Can you work these out from the drawing? Everything is in mm from the part's minimum corner. A direction names the side the tool comes from. Give positions to 0.01 mm unless a question says otherwise; leave off trailing zeros. Write each loop counter-clockwise with the first axis right and the second up, starting at its lowest first coordinate (ties: lowest second). Pieces come first, ordered by that corner, then holes. Notation, with made-up numbers: M 13,42.25 L 39,42.25 A30 ccw 39,77.25 Z; hole C -28,10.25 d7. An arc over 180 degrees is marked long. One line per item, written item: value.
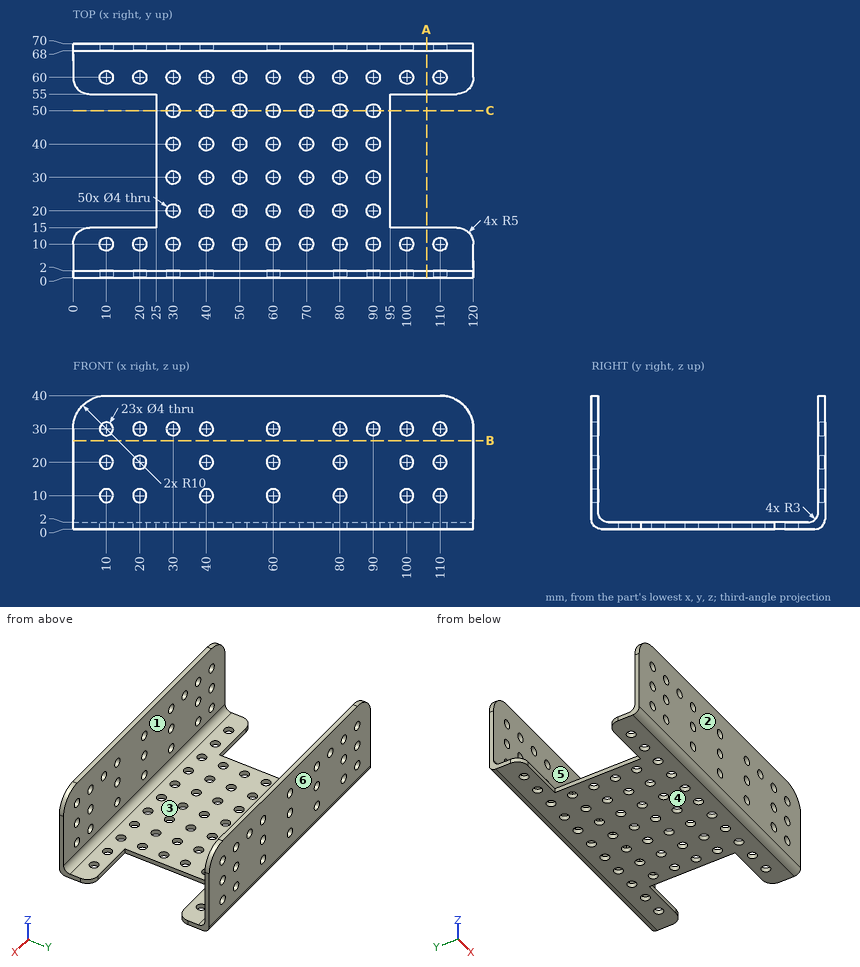
1) On a 3-axis mill with a long thin cutter (end or side, diameter ignored), from which of +Z, -Z, +X, -X, +Y, -Y can I reach the whole of each face in a straight line? I mean the marked faces 1 and 2. Say none if no direction works.
Outcome:
face 1: +Z, +X, -X
face 2: +Z, -Z, +X, -X, -Y
2) If we section it at B-B, the plane z = 26.5: Write out the boundary of the cut face in (x, y).
Outcome:
outline: M 0,0 L 120,0 L 120,2 L 0,2 Z; M 0,68 L 120,68 L 120,70 L 0,70 Z
3) Please list where these lines run through material, in increasing order: L1, parallel to Y at x = 25, z = 11.5; L2, parallel to Y at x = 10, z = 1; L3, parallel to Z at x = 92.5, y = 12. Write a range as from..to.
Outcome:
L1: y = 0..2, 68..70
L2: y = 0.76..8, 12..15, 55..58, 62..69.24
L3: z = 0..2
4) If we section it at C-C, the plane y = 50: Give the number of separate pieces and of enclosed holes in the cut face, then the cut area to 3 significant figures.
Outcome:
separate pieces: 8
enclosed holes: 0
area: 84.0 mm^2
5) We'd pull the mould along Y, two halves only. Please class the marked faces 3, 4, 5 and 6: pulls with the +Y half, pulls with the -Y half, needs draft (parallel to the pull), parting line crosses it, or undercut.
Outcome:
face 3: undercut
face 4: needs draft
face 5: undercut
face 6: pulls with the +Y half
6) If we section it at A-A, the plane x = 106: Write out the boundary of the cut face in (y, z), then the cut area to 3 significant figures.
Outcome:
outline: M 0,3 A3 ccw 3,0 L 15,0 L 15,2 L 5,2 A3 cw 2,5 L 2,40 L 0,40 Z; M 55,0 L 67,0 A3 ccw 70,3 L 70,40 L 68,40 L 68,5 A3 cw 65,2 L 55,2 Z
area: 212 mm^2
7) I'm going to push flat-ended pins straight in: pin 1 (0.6 mm diameter, centred on x = 15, z = 1, fed in from -Y); pin 2 (3 mm diameter, centred on x = 20, z = 30, fed in from -Y) (3 decimals); pin 3 (6.5 mm diameter, centred on x = 110, y = 10, fed in from +Z). Where does each tip first touch, or does it pass through?
Outcome:
pin 1: stops at y = 0.53
pin 2: passes through
pin 3: stops at z = 2
